Verification items for the finished model (mm, model axes). Round coordinates to 2 decimals unless told otherwise and drop trailing zeros. Loops run counter-clockwise (first coordinate to the right, second up) from the corner with the lowest first, then second, coordinate; pieces in that order, holes last. Notation, with made-up numbers: (-22, 41.25) - (26, 41.25) arc R23 cw to (26, 65.25) - close; hole circle Ø7 at (-7.75, 21). An arc over 180 degrees is marked (long way). Use CSV: the item, a comma, the result in double quotes.
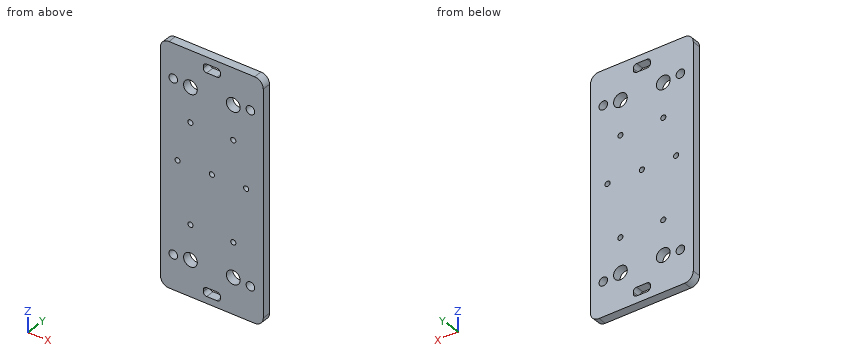
Autodesk Inventor part; units mm, degrees
ref_plane "YZ Plane" through (0, 0, 0) normal (1, 0, 0) x (0, 1, 0)
ref_plane "XZ Plane" through (0, 0, 0) normal (0, 1, 0) x (-1, 0, 0)
ref_plane "XY Plane" through (0, 0, 0) normal (0, 0, 1) x (1, 0, 0)
sketch "Sketch1" plane through (0, 0, 0) normal (0, 1, 0) x (-1, 0, 0)
  line L0 (0, 0) -> (60, 0)
  line L1 (60, 0) -> (60, -140)
  line L2 (60, -140) -> (0, -140)
  line L3 (0, -140) -> (0, 0)
  line L4 (30, -20.8594) -> (30, -183.1932) construction
  line L5 (42.5, -21.7206) -> (42.5, -191.0157) construction
  line L6 (17.5, -21.7206) -> (17.5, -184.1979) construction
  circle A0 centre (42.5, -21) radius 4
  circle A1 centre (42.5, -41) radius 1.5
  circle A2 centre (42.5, -99) radius 1.5
  circle A3 centre (42.5, -119) radius 4
  circle A4 centre (17.5, -99) radius 1.5
  circle A5 centre (17.5, -119) radius 4
  circle A6 centre (17.5, -41) radius 1.5
  circle A7 centre (17.5, -21) radius 4
  dimension "d0" = 140
  dimension "d1" = 60
  dimension "d2" = 30
  dimension "d3" = 12.5
  dimension "d4" = 12.5
  dimension "d5" = 8
  dimension "d6" = 3
  dimension "d7" = 3
  dimension "d8" = 8
  dimension "d9" = 3
  dimension "d10" = 8
  dimension "d11" = 3
  dimension "d12" = 8
  dimension "d13" = 20
  dimension "d14" = 20
  dimension "d15" = 20
  dimension "d16" = 20
  dimension "d17" = 21
  dimension "d18" = 21
  dimension "d19" = 21
  dimension "d20" = 21
extrude "Extrusion1" add sketch "Sketch1" along normal blind 5
sketch "Sketch2" plane through (0, 0, 0) normal (0, -1, 0) x (1, 0, 0)
  circle A0 centre (-52.5, -120) radius 2.5
  circle A1 centre (-52.5, -20) radius 2.5
  circle A2 centre (-7.5, -120) radius 2.5
  circle A3 centre (-7.5, -20) radius 2.5
  line L0 (-60, -140) -> (-60, 0)
  line L1 (0, -140) -> (-60, -140)
  line L2 (-60, 0) -> (0, 0)
  line L3 (0, 0) -> (0, -140)
  dimension "d23" = 5
  dimension "d24" = 5
  dimension "d25" = 5
  dimension "d26" = 5
  dimension "d27" = 7.5
  dimension "d28" = 20
  dimension "d29" = 7.5
  dimension "d30" = 20
  dimension "d31" = 20
  dimension "d32" = 7.5
  dimension "d33" = 20
  dimension "d34" = 7.5
extrude "Extrusion2" cut sketch "Sketch2" against normal blind 10 contours A0 | A1 | A2 | A3
sketch "Sketch3" plane through (0, 0, 0) normal (0, -1, 0) x (1, 0, 0)
  line L0 (-68.3542, -70) -> (15.9682, -70) construction
  line L1 (0, -140) -> (-60, -140)
  line L2 (-35, -136) -> (-25, -136)
  line L3 (-25, -136) -> (-25, -131)
  line L4 (-25, -131) -> (-35, -131)
  line L5 (-35, -131) -> (-35, -136)
  line L6 (-60, -140) -> (-60, 0)
  line L7 (-35, -4) -> (-25, -4)
  line L8 (-25, -4) -> (-25, -9)
  line L9 (-25, -9) -> (-35, -9)
  line L10 (-35, -9) -> (-35, -4)
  point P0 (0, 0)
  dimension "d40" = 70
  dimension "d41" = 10
  dimension "d42" = 25
  dimension "d43" = 4
  dimension "d44" = 5
extrude "Extrusion3" cut sketch "Sketch3" against normal blind 10
fillet "Fillet2" radius 5 4 edges at (0, 2.5, -140) (-60, 2.5, -140) (-60, 2.5, 0) (0, 2.5, 0)
sketch "Sketch4" plane through (0, 5, 0) normal (0, 1, 0) x (1, 0, 0)
  circle A0 centre (-10, 65.5) radius 1.5
  circle A1 centre (-30, 65.5) radius 1.5
  circle A2 centre (-50, 65.5) radius 1.5
  line L0 (3.8133, 65.5) -> (-51.9818, 65.5) construction
  line L1 (-55, 0) -> (-5, 0)
  line L2 (0, 5) -> (0, 135)
  point P0 (0, 0)
  dimension "d49" = 3
  dimension "d50" = 3
  dimension "d51" = 3
  dimension "d52" = 65.5
  dimension "d53" = 10
  dimension "d54" = 30
  dimension "d55" = 50
extrude "Extrusion4" cut sketch "Sketch4" against normal blind 10
fillet "Fillet3" radius 2 8 edges at (-25, 2.5, -131) (-25, 2.5, -136) (-35, 2.5, -136) (-35, 2.5, -131) (-25, 2.5, -9) (-25, 2.5, -4) (-35, 2.5, -4) (-35, 2.5, -9)
equation "\"d2\" = 0.5 * d1"
equation "\"d4\" = d3"
equation "\"d8\" = d5"
equation "\"d10\" = d5"
equation "\"d12\" = d5"
equation "\"d14\" = d13"
equation "\"d15\" = d13"
equation "\"d16\" = d13"
equation "\"d18\" = d17"
equation "\"d19\" = d17"
equation "\"d20\" = d17"
equation "\"d29\" = d27"
equation "\"d30\" = d28"
equation "\"d31\" = d28"
equation "\"d32\" = d27"
equation "\"d33\" = d28"
equation "\"d34\" = d27"
properties part number "Y-Axis_back_plate_top" material "PET Plastic"
1) Cross-section at B-B, the plane x = -42.5. Record the cut outline in (y, z), then the cut area to 3 significant figures.
Returned:
outline,"(0, -140) - (5, -140) - (5, -123) - (0, -123) - close; (0, -115) - (5, -115) - (5, -100.5) - (0, -100.5) - close; (0, -97.5) - (5, -97.5) - (5, -42.5) - (0, -42.5) - close; (0, -39.5) - (5, -39.5) - (5, -25) - (0, -25) - close; (0, -17) - (5, -17) - (5, 0) - (0, 0) - close"
area,"590 mm²"
2) Thickness scan on probe 1 along Z at (x, y) = (-52.5, 2.05); probe 2 along Z at (x, y) = (-42.5, 3.75); probe 3 along Z at (x, y) = (-30, 3.35). Record the ranges inside material, lowest first. Write a range as [from, to].
Returned:
probe 1,"z = [-140, -122.5], [-117.5, -22.5], [-17.5, 0]"
probe 2,"z = [-140, -123], [-115, -100.5], [-97.5, -42.5], [-39.5, -25], [-17, 0]"
probe 3,"z = [-140, -136], [-131, -67], [-64, -9], [-4, 0]"
3) Cross-section at D-D, the plane y = 2.85. Count the separate pieces of the cut face and the enclosed holes in it, then the cut area to 3 significant figures.
Returned:
separate pieces,"1"
enclosed holes,"17"
area,"7,960 mm²"
4) Cross-section at C-C, the plane z = -65.5. Record the cut outline in (x, y), then the cut area to 3 significant figures.
Returned:
outline,"(-60, 0) - (-51.5, 0) - (-51.5, 5) - (-60, 5) - close; (-48.5, 0) - (-31.5, 0) - (-31.5, 5) - (-48.5, 5) - close; (-28.5, 0) - (-11.5, 0) - (-11.5, 5) - (-28.5, 5) - close; (-8.5, 0) - (0, 0) - (0, 5) - (-8.5, 5) - close"
area,"255 mm²"
5) Cross-section at A-A, the plane z = -41. Record the cut outline in (x, y).
Returned:
outline,"(-60, 0) - (-44, 0) - (-44, 5) - (-60, 5) - close; (-41, 0) - (-19, 0) - (-19, 5) - (-41, 5) - close; (-16, 0) - (0, 0) - (0, 5) - (-16, 5) - close"
6) Gauge pin test, flat ends, axial feed: pin 1 Ø2.5 at (x, z) = (-17.5, -99) entering from +Y; pin 2 Ø6 at (x, z) = (-52.5, -120) entering from +Y. Record the tip position at first contact, or that the pin passes through.
Returned:
pin 1,"passes through"
pin 2,"stops at y = 5"
